Input: part model. Units: mm. Frame: model coordinates. Face numbers are marked on the shaded views. A direction names the side the tool comes from. Give positions to 0.01 mm unless a question says otherwise; leave off trailing zeros. Loops run counter-clockwise (first coordinate to the right, second up) from the corner with the lowest first, then second, coordinate; pieces in that order, holes last. Notation, with made-up numbers: (29, -10.5) -> (52, -10.5) arc R4 ccw to (52, -4.5) -> close; hole circle Ø6 at (23.25, 17.5). An arc over 180 degrees is marked (long way). One line per question, with ' | ' between items.
Autodesk Inventor part; units mm, degrees
ref_plane "YZ Plane" through (0, 0, 0) normal (1, 0, 0) x (0, 1, 0)
ref_plane "XZ Plane" through (0, 0, 0) normal (0, 1, 0) x (-1, 0, 0)
ref_plane "XY Plane" through (0, 0, 0) normal (0, 0, 1) x (1, 0, 0)
sketch "スケッチ1" plane through (0, 0, 0) normal (0, 0, 1) x (1, 0, 0)
  line L0 (0, 0) -> (0, 64)
  line L1 (0, 32) -> (75, 32) construction
  line L2 (0, 0) -> (9, 0)
  line L3 (9, 0) -> (9, 12)
  line L4 (9, 12) -> (15, 12)
  line L5 (15, 12) -> (32, 29)
  line L6 (32, 29) -> (52, 29)
  line L7 (52, 29) -> (52, 12)
  line L8 (52, 12) -> (75, 12)
  line L9 (75, 12) -> (75, 32)
  line L10 (0, 64) -> (9, 64)
  line L11 (9, 64) -> (9, 52)
  line L12 (9, 52) -> (15, 52)
  line L13 (15, 52) -> (32, 35)
  line L14 (32, 35) -> (52, 35)
  line L15 (52, 35) -> (52, 52)
  line L16 (52, 52) -> (75, 52)
  line L17 (75, 52) -> (75, 32)
  dimension "d0" = 9
  dimension "d1" = 12
  dimension "d3" = 3
  dimension "d6" = 20
  dimension "d7" = 135
  dimension "d8" = 75
  dimension "d9" = 20
  dimension "d10" = 20
  dimension "d14" = 15
revolve "回転1" add sketch "スケッチ1" angle 360 about axis through (0, 0, 0) along (0, 1, 0)
fillet "フィレット1" radius 5 2 edges at (-75, 12, 0) (-75, 52, 0)
fillet "フィレット2" radius 5 2 edges at (-52, 12, 0) (-52, 52, 0)
properties part number "自由輪パーツ3"
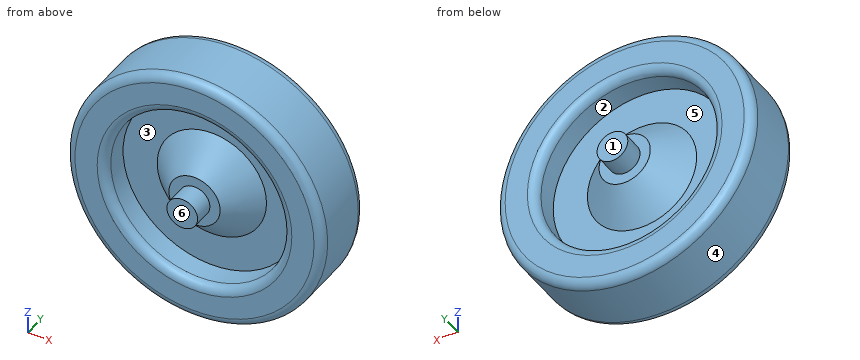
1. Ray query, line 1 along Z through (x, y) = (0, 24.75); line 2 along Z through (x, y) = (0, 23); line 3 along X through (y, z) = (43, -10). Return the intervals inside material, ascending. Write a range as from..to.
Determined:
line 1: z = -75..-52, -27.75..27.75, 52..75 | line 2: z = -75..-52, -26..26, 52..75 | line 3: x = -74.33..-51.03, -21.82..21.82, 51.03..74.33
2. Pull-direction query (X, two-part tool) for the marked faces 4, 5 and 6; classes: pulls with the +X half, pulls with the -X half, needs draft (parallel to the pull), parting line crosses it, or undercut.
Determined:
face 4: parting line crosses it | face 5: undercut | face 6: needs draft
3. Section query A-A (y = 43). Output: boundary loops of the cut face in (x, z), then the cut area to 3 significant figures.
Determined:
outline: circle Ø150 at (0, 0); circle Ø48 at (0, 0); hole circle Ø104 at (0, 0) | area: 11,000 mm2
4. Reachability of the marked faces 1, 2 and 3 from +Z, -Z, +X, -X, +Y, -Y: full face, straight path, thin tool, end or side. Return the list, or none.
Determined:
face 1: +Z, -Z, +X, -X, +Y | face 2: +Y | face 3: -Y
5. Section query B-B (y = 9.5). Output: boundary loops of the cut face in (x, z), then the cut area to 3 significant figures.
Determined:
outline: circle Ø18 at (0, 0) | area: 254 mm2
6. Pin query (flat end, axial travel): P1, Ø12, axis at y = 22, z = -16, coming from the -X side; P2, Ø1.5, axis at y = 22, z = -29, coming from the +X side; P3, Ø3, axis at x = 49.5, z = -34, coming from the +Y side. Return the tip coordinate at first contact, or that it passes through.
Determined:
P1: stops at x = -74.33 | P2: stops at x = 69.48 | P3: stops at y = 52
